Read the model definition and answer for the solid it produces. Units are mm, in the model's axes. Give positions to 0.01 mm unless a question says otherwise; leave off trailing zeros. Write each loop counter-clockwise with the first axis right and the second up, starting at its lowest first coordinate (ties: lowest second). Pieces come first, ordered by that corner, then holes. Notation, with made-up numbers: M -26.5,83 L 27.5,83 A28 cw 27.5,111 Z; hole C -37.5,73 d7. An arc over 180 degrees is marked long. Put each result on its own line as item: value.
from build123d import *

# Parameters (mm, degrees)
SKETCH1_W                 = 160
SKETCH1_H                 = 140
BOSS_EXTRUDE1_DEPTH       = 80
F_3_0MM_DOWEL_HOLE3_D     = 3
SHELL1_T                  = -2
SKETCH10_R                = 2.5
BOSS_EXTRUDE3_DEPTH       = 60
F_3_0MM_DOWEL_HOLE2_D     = 3
F_3_0MM_DOWEL_HOLE2_DEPTH = 45
F_3_0MM_DOWEL_HOLE2_TIP   = 0.901290929
FILLET1_R                 = 4
SKETCH15_R                = 2.5
BOSS_EXTRUDE5_DEPTH       = 10
F_3_0MM_DOWEL_HOLE5_D     = 3
SKETCH20_W                = 13
SKETCH20_H                = 20
CUT_EXTRUDE1_DEPTH        = 2
F_5_0MM_DOWEL_HOLE1_D     = 5
F_5_0MM_DOWEL_HOLE1_DEPTH = 2
SKETCH27_W                = 10
SKETCH27_H                = 11.5
CUT_EXTRUDE2_DEPTH        = 2


with BuildPart() as part:
    # Sketch1 → Boss-Extrude1 (new body)
    with BuildSketch(Plane(origin=(0, 0, 0), x_dir=(1, 0, 0), z_dir=(0, 1, 0))):
        Rectangle(SKETCH1_W, SKETCH1_H)
    extrude(amount=BOSS_EXTRUDE1_DEPTH)

    # Ø3.0mm Dowel Hole3 (through all)
    with Locations(Plane(origin=(0, 80, 0), x_dir=(1, 0, 0), z_dir=(0, 1, 0))):
        with Locations((-76, 66), (76, 66), (76, -66), (-76, -66)):
            Hole(F_3_0MM_DOWEL_HOLE3_D / 2)

    # Shell1
    shell1_openings = [part.faces().sort_by_distance(p)[0] for p in [
        (-76, 80, -64.5),
    ]]
    offset(amount=SHELL1_T, openings=shell1_openings, kind=Kind.INTERSECTION)

    # Sketch10 → Boss-Extrude3 (add)
    with BuildSketch(Plane(origin=(0, 2, 0), x_dir=(1, 0, 0), z_dir=(0, 1, 0))):
        with Locations((70, 46.925)):
            Circle(SKETCH10_R)
        with Locations((-23.85, 46.925)):
            Circle(SKETCH10_R)
        with Locations((-23.85, -46.925)):
            Circle(SKETCH10_R)
        with Locations((70, -46.925)):
            Circle(SKETCH10_R)
    extrude(amount=BOSS_EXTRUDE3_DEPTH)

    # Ø3.0mm Dowel Hole2
    with Locations(Plane(origin=(0, 62, 0), x_dir=(1, 0, 0), z_dir=(0, 1, 0))):
        with Locations((-23.85, 46.925), (70, 46.925), (70, -46.925), (-23.85, -46.925)):
            Hole(F_3_0MM_DOWEL_HOLE2_D / 2, depth=F_3_0MM_DOWEL_HOLE2_DEPTH)
            with Locations((0, 0, -(F_3_0MM_DOWEL_HOLE2_DEPTH + F_3_0MM_DOWEL_HOLE2_TIP / 2))):  # 118° drill point
                Cone(0, F_3_0MM_DOWEL_HOLE2_D / 2, F_3_0MM_DOWEL_HOLE2_TIP, mode=Mode.SUBTRACT)

    # Fillet1
    fillet1_edges = [part.edges().sort_by_distance(p)[0] for p in [
        (78, 41, 63.127718677),
        (73.127718677, 41, -68),
        (-78, 41, -63.127718677),
        (-73.127718677, 41, 68),
        (-78, 41, 63.127718677),
        (73.127718677, 41, 68),
        (78, 41, -63.127718677),
        (-73.127718677, 41, -68),
    ]]
    fillet(fillet1_edges, radius=FILLET1_R)

    # Sketch15 → Boss-Extrude5 (add)
    with BuildSketch(Plane(origin=(0, 2, 0), x_dir=(1, 0, 0), z_dir=(0, 1, 0))):
        with Locations((-3.85, 26.925)):
            Circle(SKETCH15_R)
        with Locations((50, 26.925)):
            Circle(SKETCH15_R)
        with Locations((-3.85, -26.925)):
            Circle(SKETCH15_R)
        with Locations((50, -26.925)):
            Circle(SKETCH15_R)
    extrude(amount=BOSS_EXTRUDE5_DEPTH)

    # Ø3.0mm Dowel Hole5 (through all)
    with Locations(Plane(origin=(0, 12, 0), x_dir=(1, 0, 0), z_dir=(0, 1, 0))):
        with Locations((-3.85, 26.925), (50, 26.925), (50, -26.925), (-3.85, -26.925)):
            Hole(F_3_0MM_DOWEL_HOLE5_D / 2)

    # Sketch20 → Cut-Extrude1 (cut)
    with BuildSketch(Plane.XY.offset(70)):
        with Locations((-56.5, 50)):
            Rectangle(SKETCH20_W, SKETCH20_H)
    extrude(amount=-CUT_EXTRUDE1_DEPTH, mode=Mode.SUBTRACT)

    # Ø5.0mm Dowel Hole1
    with Locations(Plane.XY.offset(70)):
        with Locations((-15, 30), (5, 30)):
            Hole(F_5_0MM_DOWEL_HOLE1_D / 2, depth=F_5_0MM_DOWEL_HOLE1_DEPTH)

    # Sketch27 → Cut-Extrude2 (cut)
    with BuildSketch(Plane(origin=(0, 0, -70), x_dir=(-1, 0, 0), z_dir=(0, 0, -1))):
        with Locations((55, 20.75)):
            Rectangle(SKETCH27_W, SKETCH27_H)
    extrude(amount=-CUT_EXTRUDE2_DEPTH, mode=Mode.SUBTRACT)


solid = part.part
(1) Section A-A on x = -15 is taken. Determine the outline of the cut face in (y, z), and give its area (3 significant figures).
Result:
outline: M 0,-70 L 80,-70 L 80,-68 L 2,-68 L 2,68 L 27.5,68 L 27.5,70 L 0,70 Z; M 32.5,68 L 80,68 L 80,70 L 32.5,70 Z
area: 582 mm²
(2) Section D-D on x = 40.5 is taken. Determine the outline of the cut face in (y, z).
Result:
outline: M 0,-70 L 80,-70 L 80,-68 L 2,-68 L 2,68 L 80,68 L 80,70 L 0,70 Z
(3) For a pull along Z with two mould halves and no side action, classify faces 1 (the face through (-13.16, 31.69, 68.99)), 2 (the face through (71.223, 40.454, 67.161)), 3 (the face through (-1, 39, 70)) as +Z half, -Z half, draft (parallel to the pull), parting line (faces both ways), or undercut.
Result:
face 1: draft
face 2: undercut
face 3: +Z half
(4) Section B-B on y = 35 is taken. Give the number of separate pieces and of enclosed holes in the cut face, and give its area (3 significant figures).
Result:
separate pieces: 5
enclosed holes: 9
area: 1,340 mm²
(5) Section C-C on z = 13 is taken. Determine the outline of the cut face in (x, y).
Result:
outline: M -80,0 L 80,0 L 80,80 L 78,80 L 78,2 L -78,2 L -78,80 L -80,80 Z
(6) Straight lines are drawn through the part: line 1 along Z through (x, y) = (-3.85, 7.25) (3 decimals); line 2 along X through (y, z) = (65, 59); line 3 along Z through (x, y) = (-24, 14.5). For each, find the intervals that lie inside material, in ascending order. Write a range as from..to.
Result:
line 1: z = -70..-68, -29.425..-28.425, -25.425..-24.425, 24.425..25.425, 28.425..29.425, 68..70
line 2: x = -80..-77.99, 77.99..80
line 3: z = -70..-68, -49.42..-44.43, 44.43..49.42, 68..70
(7) Given pin 1 Ø2.5 at (x, z) = (71, -46) entering from +Y; pin 2 Ø4 at (x, z) = (50, -27) entering from +Y, each flat-ended and moving along its own axis, determine where each tip first touches the part or whether it passes through.
Result:
pin 1: stops at y = 62
pin 2: stops at y = 12
